```python
from build123d import *

# Parameters (mm, degrees)
SKETCH_1_R      = 1.5
EXTRUDE_1_DEPTH = 3


with BuildPart() as part:
    # 草圖1 → 填料-伸長1 (new body)
    with BuildSketch(Plane(origin=(0, 3, 0), x_dir=(1, 0, 0), z_dir=(0, 1, 0))):
        with BuildLine():
            Line((-46, 43), (-46, -43))
            ThreePointArc((-46, -43), (-45.121320344, -45.121320344), (-43, -46))
            Line((-43, -46), (43, -46))
            ThreePointArc((43, -46), (45.121320344, -45.121320344), (46, -43))
            Line((46, -43), (46, 43))
            ThreePointArc((46, 43), (45.121320344, 45.121320344), (43, 46))
            Line((43, 46), (-43, 46))
            ThreePointArc((-43, 46), (-45.121320344, 45.121320344), (-46, 43))
        make_face()
        with Locations((-29.285, 36.6)):
            Circle(SKETCH_1_R, mode=Mode.SUBTRACT)
        with Locations((32.435, 36.6)):
            Circle(SKETCH_1_R, mode=Mode.SUBTRACT)
        with Locations((32.435, -40)):
            Circle(SKETCH_1_R, mode=Mode.SUBTRACT)
        with Locations((-29.285, -40)):
            Circle(SKETCH_1_R, mode=Mode.SUBTRACT)
        with Locations((41.25, -41.25)):
            Circle(SKETCH_1_R, mode=Mode.SUBTRACT)
        with Locations((-41.25, 41.25)):
            Circle(SKETCH_1_R, mode=Mode.SUBTRACT)
        with Locations((41.25, 41.25)):
            Circle(SKETCH_1_R, mode=Mode.SUBTRACT)
        with Locations((-41.25, -41.25)):
            Circle(SKETCH_1_R, mode=Mode.SUBTRACT)
        Polygon((-19.285, 36.6), (22.435, 36.6), (32.435, 26.6), (32.435, -30), (22.435, -40), (-19.285, -40), (-29.285, -30), (-29.285, 26.6), align=None, mode=Mode.SUBTRACT)
    extrude(amount=-EXTRUDE_1_DEPTH)


solid = part.part
```
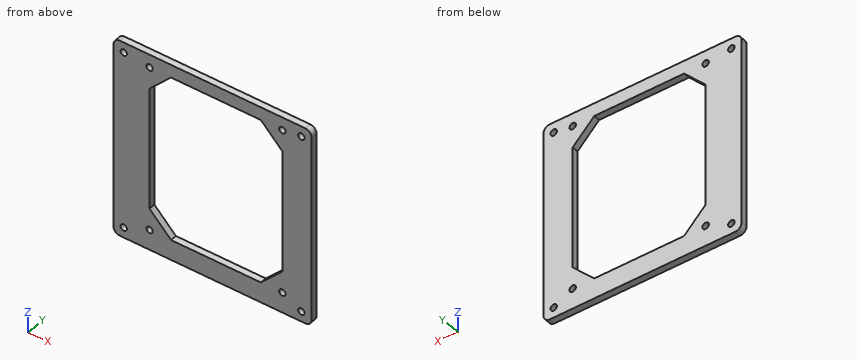
Verification items for the finished model (mm, model axes). Round coordinates to 2 decimals unless told otherwise and drop trailing zeros. Order: outer loops, then holes, each group sorted by start corner. A loop starts at its lowest first (then second) coordinate and runs counter-clockwise, first axis right, second up. Notation, with made-up numbers: (-28.5, -17) -> (13.5, -17) arc R11 ccw to (13.5, -1) -> close; hole circle Ø8 at (54, -14.75). An arc over 180 degrees is marked (long way). Put each result on its own line as item: value. Start each with the question number.
(1) Material ranges on line 1 along X through (y, z) = (1.25, -41.25); line 2 along Z through (x, y) = (41, 2.45); line 3 along X through (y, z) = (0.95, -12.5) (3 decimals), recorded low to high.
(2) Section check A-A (x = -12.5). Enter the section's corners in (y, z).
(3) Section check C-C (x = -41.25). Enter the section's corners in (y, z).
(4) Section check B-B (y = 2.5). State how many separate pieces and enclosed holes the cut face has, then the cut area to 3 significant figures.
(5) Section check D-D (z = 35). Enter the section's corners in (x, y) (3 decimals), then the cut area to 3 significant figures.
Completed:
1. line 1: x = -46 to -42.75, -39.75 to 39.75, 42.75 to 46
1. line 2: z = -46 to -42.73, -39.77 to 39.77, 42.73 to 46
1. line 3: x = -46 to -29.285, 32.435 to 46
2. outline: (0, -46) -> (3, -46) -> (3, -36.6) -> (0, -36.6) -> close; (0, 40) -> (3, 40) -> (3, 46) -> (0, 46) -> close
3. outline: (0, -46) -> (3, -46) -> (3, -42.75) -> (0, -42.75) -> close; (0, -39.75) -> (3, -39.75) -> (3, 39.75) -> (0, 39.75) -> close; (0, 42.75) -> (3, 42.75) -> (3, 46) -> (0, 46) -> close
4. separate pieces: 1
4. enclosed holes: 9
4. area: 3,870 mm2
5. outline: (-46, 0) -> (-24.285, 0) -> (-24.285, 3) -> (-46, 3) -> close; (27.435, 0) -> (46, 0) -> (46, 3) -> (27.435, 3) -> close
5. area: 121 mm2
